Here's how the part is built. I have some questions about the finished solid (model axes, mm). Face numbers are marked on the shaded views. A direction names the side the tool comes from. Coordinates: 2 decimals unless noted, no trailing zeros. Write each loop counter-clockwise with the first axis right and the second up, starting at its lowest first coordinate (ties: lowest second). Pieces come first, ordered by that corner, then holes.
Item 1: If we section it at C-C (z = 3): Please give me the cut outline in (x, y), then the cut area to 3 significant figures.
Item 2: If we section it at D-D (y = -2.75): Please give me the cut outline in (x, z), then the cut area to 3 significant figures.
Item 3: If I drill on line 1 (Z direction, x = -1.5, y = 1.5); line 2 (X direction, y = -1.5, z = -7); line 3 (Z direction, x = -0.25, y = 1.5), over which ranges is the centre line in solid material (lowest first)?
Item 4: If we section it at A-A (x = 0): Please give me the cut outline in (y, z).
Item 5: For the marked faces 1, 2 and 3, which set-ups out of +Z, -Z, +X, -X, +Y, -Y let a thin tool reach every point of the face, with its end or its side?
Item 6: I'm going to push flat-ended pins straight in: pin 1 Ø3 at (x, z) = (-2.5, -2.5) entering from +Y; pin 2 Ø1.5 at (x, y) = (-1.5, 2) entering from -Z; pin 3 Ø1.5 at (x, y) = (2, -2.5) entering from +Z; pin 4 Ø3 at (x, z) = (3, -6) entering from +Y. Where does each tip first touch, or does it pass through?
from build123d import *

# Parameters (mm, degrees)
F0_R     = 2
F1_DEPTH = 10
F2_R     = 4
F3_DEPTH = 1
F4_R     = 2
F5_DEPTH = 17
F6_R     = 1.8
F7_DEPTH = 0.5
F8_R     = 2
F8_R_2   = 1.8
F9_DEPTH = 1
F10_SIZE = 0.6


with BuildPart() as f1:
    # F0 (on Top) → F1 (new body)
    with BuildSketch(Plane.XY):
        Circle(F0_R)
    extrude(amount=-F1_DEPTH)

    # F2 (on Top) → F3 (join)
    with BuildSketch(Plane.XY):
        Circle(F2_R)
    extrude(amount=F3_DEPTH)

    # F4 (on face) → F5 (join)
    with BuildSketch(Plane.XY.offset(1)):
        Circle(F4_R)
    extrude(amount=F5_DEPTH)

    # F6 (on face) → F7 (join)
    with BuildSketch(Plane.XY.offset(18)):
        Circle(F6_R)
    extrude(amount=F7_DEPTH)

    # F8 (on face) → F9 (join)
    with BuildSketch(Plane.XY.offset(18.5)):
        Circle(F8_R)
        Circle(F8_R_2, mode=Mode.SUBTRACT)
        Circle(F8_R_2)
    extrude(amount=F9_DEPTH)

    # F10
    f10_edges = [f1.edges().sort_by_distance(p)[0] for p in [
        (-2, 0, 19.5),
    ]]
    chamfer(f10_edges, length=F10_SIZE)


solid = f1.part
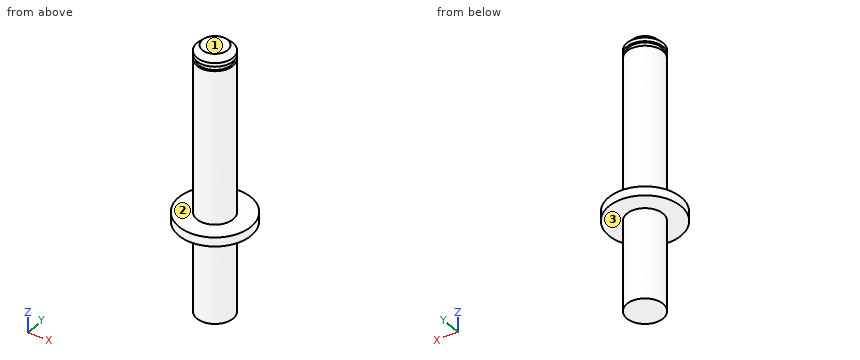
Answer list:
1. outline: circle Ø4 at (0, 0)
1. area: 12.6 mm2
2. outline: (-2.9, 0) - (2.9, 0) - (2.9, 1) - (-2.9, 1) - close
2. area: 5.81 mm2
3. line 1: z = 0 to 1
3. line 2: x = -1.32 to 1.32
3. line 3: z = -10 to 19.38
4. outline: (-4, 0) - (-2, 0) - (-2, -10) - (2, -10) - (2, 0) - (4, 0) - (4, 1) - (2, 1) - (2, 18) - (1.8, 18) - (1.8, 18.5) - (2, 18.5) - (2, 18.9) - (1.4, 19.5) - (-1.4, 19.5) - (-2, 18.9) - (-2, 18.5) - (-1.8, 18.5) - (-1.8, 18) - (-2, 18) - (-2, 1) - (-4, 1) - close
5. face 1: +Z, +X, -X, +Y, -Y
5. face 2: +Z
5. face 3: -Z
6. pin 1: stops at y = 1.73
6. pin 2: stops at z = -10
6. pin 3: stops at z = 1
6. pin 4: stops at y = 1.32
